Input: part model. Units: mm. Frame: model coordinates. A direction names the side the tool comes from. Round coordinates to 2 decimals unless told otherwise and drop trailing zeros. Order: outer loops, then holes, each group sorted by start corner. A loop starts at its lowest first (then second) coordinate and runs counter-clockwise, first axis right, second up. Notation, with made-up numbers: (43, 20.25) -> (72, 20.25) arc R22 ccw to (72, 32.25) -> close; hole circle Ø9 at (56, 33). An arc over 180 degrees is marked (long way). Answer as CSV lines item,"result". Start each with the question number.
1) Line query: L1, parallel to Z at x = 192, y = 7.5; L2, parallel to Z at x = 180, y = 17.5; L3, parallel to X at y = 8, z = -10. Output: solid intervals per line, ascending.
2) Section query C-C, the plane y = 9.75. State how many separate pieces and enclosed holes the cut face has, and give its area (3 significant figures).
3) First-contact query: P1, Ø1.5, axis at x = 94, z = -33, coming from the +Y side. Flat tip, straight axial feed; report the tip coordinate or a pass-through.
4) Access query for faces 4 (the face through (199.5, 13, -53)), 5 (the face through (108, 10, -65)). Directions: +Z, -Z, +X, -X, +Y, -Y. A direction counts if a zero-diameter tool reaches every point of the face in a straight line with its end or side. Return the directions, or none.
5) Section query A-A, the plane z = -48. Output: boundary loops of the cut face in (x, y).
6) Mould query, pull axis X, two halves, no side actions, for faces 1 (the face through (0, 10, -32)), 2 (the face through (24.5, 13, -53)), 3 (the face through (116, 5, -32)). Classes: +X half, -X half, draft (parallel to the pull), parting line (faces both ways), or undercut.
7) Section query B-B, the plane x = 57.5. Output: boundary loops of the cut face in (y, z).
```python
from build123d import *

# Parameters (mm, degrees)
SKICA1_W                 = 220
SKICA1_H                 = 65
P_IDAT_VYSUNUT_M1_DEPTH  = 20
SKICA2_W                 = 200
SKICA2_H                 = 5
ODEBRAT_VYSUNUT_M1_DEPTH = 15
SKICA3_W                 = 5
SKICA3_H                 = 7
ODEBRAT_VYSUNUT_M2_DEPTH = 35


with BuildPart() as part:
    # Skica1 → Přidat vysunutím1 (new body)
    with BuildSketch(Plane(origin=(0, 0, 0), x_dir=(1, 0, 0), z_dir=(0, 1, 0))):
        with Locations((110, 32.5)):
            Rectangle(SKICA1_W, SKICA1_H)
    extrude(amount=P_IDAT_VYSUNUT_M1_DEPTH)

    # Skica2 → Odebrat vysunutím1 (cut)
    with BuildSketch(Plane(origin=(0, 20, 0), x_dir=(1, 0, 0), z_dir=(0, 1, 0))):
        with Locations((110, 32.5)):
            Rectangle(SKICA2_W, SKICA2_H)
        Polygon((24.5, 50), (30, 50), (30, 46), (24.5, 46), (24.5, 40.5), (20.5, 40.5), (20.5, 46), (15, 46), (15, 50), (20.5, 50), (20.5, 55.5), (24.5, 55.5), align=None)
        Polygon((15, 15), (15, 19), (20.5, 19), (20.5, 24.5), (24.5, 24.5), (24.5, 19), (30, 19), (30, 15), (24.5, 15), (24.5, 9.5), (20.5, 9.5), (20.5, 15), align=None)
        Polygon((205, 15), (199.5, 15), (199.5, 9.5), (195.5, 9.5), (195.5, 15), (190, 15), (190, 19), (195.5, 19), (195.5, 24.5), (199.5, 24.5), (199.5, 19), (205, 19), align=None)
        Polygon((205, 50), (205, 46), (199.5, 46), (199.5, 40.5), (195.5, 40.5), (195.5, 46), (190, 46), (190, 50), (195.5, 50), (195.5, 55.5), (199.5, 55.5), (199.5, 50), align=None)
    extrude(amount=-ODEBRAT_VYSUNUT_M1_DEPTH, mode=Mode.SUBTRACT)

    # Skica3 → Odebrat vysunutím2 (cut)
    with BuildSketch(Plane(origin=(220, 0, 0), x_dir=(0, 0, -1), z_dir=(1, 0, 0))):
        with Locations((32.5, 8.5)):
            Rectangle(SKICA3_W, SKICA3_H)
    extrude(amount=-ODEBRAT_VYSUNUT_M2_DEPTH, mode=Mode.SUBTRACT)


solid = part.part
```
Findings:
1,L1,"z = -65 to -50, -46 to -35, -30 to -19, -15 to 0"
1,L2,"z = -65 to -35, -30 to 0"
1,L3,"x = 0 to 20.5, 24.5 to 195.5, 199.5 to 220"
2,separate pieces,"1"
2,enclosed holes,"4"
2,area,"12,800 mm^2"
3,P1,"stops at y = 5"
4,face 4,"+Y"
4,face 5,"-Z, +X, -X, +Y, -Y"
5,outline,"(0, 0) -> (220, 0) -> (220, 20) -> (205, 20) -> (205, 5) -> (190, 5) -> (190, 20) -> (30, 20) -> (30, 5) -> (15, 5) -> (15, 20) -> (0, 20) -> close"
6,face 1,"-X half"
6,face 2,"undercut"
6,face 3,"draft"
7,outline,"(0, -65) -> (20, -65) -> (20, -35) -> (5, -35) -> (5, -30) -> (20, -30) -> (20, 0) -> (0, 0) -> close"
